Verification items for the finished model (mm, model axes). Give positions to 0.01 mm unless a question says otherwise; leave off trailing zeros. Order: outer loops, then holes, each group sorted by start corner. A loop starts at its lowest first (then second) coordinate and runs counter-clockwise, first axis right, second up. Notation, with made-up numbers: (39, 61.5) -> (55, 61.5) arc R20 cw to (55, 95.5) -> close; hole circle Ø8 at (34, 53.25). An arc over 180 degrees is marked (long way). Write each question's results on one line, items separated by ' | '. Start each with the question number.
1. Cross-section at A-A, the plane x = -25. Enter the section's corners in (y, z).
2. Cross-section at D-D, the plane y = -55. Enter the section's corners in (x, z), then the cut area to 3 significant figures.
3. Cross-section at C-C, the plane z = 3.85. State how many separate pieces and enclosed holes the cut face has, then the cut area to 3 significant figures.
4. Mould release check, pull along Y, two halves, no side actions. Record for faces 1 (the face through (-1, -75, 2)), 2 (the face through (-23.43, -0.65, 2.53)), 3 (the face through (-75, -1, 2)): +Y half, -Y half, draft (parallel to the pull), parting line (faces both ways), or undercut.
5. Material ranges on L1, parallel to Y at x = 0, z = 1.95; L2, parallel to X at y = 43, z = 3.3; L3, parallel to X at y = 44, z = 4.3, recorded low to high. Write a range as from..to.
from build123d import *

# Parameters (mm, degrees)
ESQUISSE1_W                  = 150
ESQUISSE1_H                  = 150
BOSS_EXTRU_1_DEPTH           = 5
ENL_V_MAT_EXTRU_1_DEPTH      = 5
D_GAGEMENT_M31_D             = 3.4
CONG_1_R                     = 0.5
ENL_V_MAT_EXTRU_2_REACH      = 108.184
ESQUISSE6_R                  = 2.75
R_P_TITION_CIRCULAIRE1_COUNT = 4


with BuildPart() as part:
    # Esquisse1 → Boss.-Extru.1 (new body)
    with BuildSketch(Plane.XY):
        Rectangle(ESQUISSE1_W, ESQUISSE1_H)
    extrude(amount=BOSS_EXTRU_1_DEPTH)

    # Esquisse2 → Enlèv. mat.-Extru.1 (cut)
    with BuildSketch(Plane.XY.offset(5)):
        with BuildLine():
            Line((45, 75), (75, 75))
            Line((75, 75), (75, 45))
            ThreePointArc((75, 45), (53.786796564, 53.786796564), (45, 75))
        make_face()
        with BuildLine():
            Line((75, -75), (45, -75))
            ThreePointArc((45, -75), (53.786796564, -53.786796564), (75, -45))
            Line((75, -45), (75, -75))
        make_face()
        with BuildLine():
            Line((-75, -75), (-75, -45))
            ThreePointArc((-75, -45), (-53.786796564, -53.786796564), (-45, -75))
            Line((-45, -75), (-75, -75))
        make_face()
        with BuildLine():
            Line((-75, 75), (-45, 75))
            ThreePointArc((-45, 75), (-53.786796564, 53.786796564), (-75, 45))
            Line((-75, 45), (-75, 75))
        make_face()
    extrude(amount=-ENL_V_MAT_EXTRU_1_DEPTH, mode=Mode.SUBTRACT)

    # Dégagement M31 (through all)
    with Locations(Plane(origin=(0, 0, 0), x_dir=(-1, 0, 0), z_dir=(0, 0, -1))):
        with Locations((0, 25), (0, -25), (60, 0), (25, 0), (-25, 0), (-60, 0)):
            Hole(D_GAGEMENT_M31_D / 2)

    # Congé1
    cong_1_edges = [part.edges().sort_by_distance(p)[0] for p in [
        (-75, 45, 2.5),
        (-45, 75, 2.5),
        (-45, -75, 2.5),
        (-75, -45, 2.5),
        (75, -45, 2.5),
        (45, -75, 2.5),
        (75, 45, 2.5),
        (45, 75, 2.5),
    ]]
    fillet(cong_1_edges, radius=CONG_1_R)

    # Esquisse6 → Enlèv. mat.-Extru.2 (cut, up to next)
    with BuildSketch(Plane(origin=(0, 0, 0), x_dir=(-1, 0, 0), z_dir=(0, 0, -1)), mode=Mode.PRIVATE) as enl_v_mat_extru_2_sk1:
        with Locations((-44.504098636, 44.504098636)):
            Circle(ESQUISSE6_R)
    enl_v_mat_extru_2_tool1 = extrude(enl_v_mat_extru_2_sk1.sketch, amount=-ENL_V_MAT_EXTRU_2_REACH, mode=Mode.PRIVATE) & part.part
    enl_v_mat_extru_2 = enl_v_mat_extru_2_tool1.solids().sort_by_distance((44.504099, 44.504099, 0))[0]
    add(enl_v_mat_extru_2, mode=Mode.SUBTRACT)

    # Répétition circulaire1: Enlèv. mat.-Extru.2 ×4 about axis
    r_p_tition_circulaire1_axis = Axis((-0.053962748, -0.053962748, 0), (0, 0, 1))
    for i in range(1, R_P_TITION_CIRCULAIRE1_COUNT):
        add(enl_v_mat_extru_2.rotate(r_p_tition_circulaire1_axis, i * 360 / R_P_TITION_CIRCULAIRE1_COUNT), mode=Mode.SUBTRACT)


solid = part.part
Results below:
1) outline: (-75, 0) -> (-1.7, 0) -> (-1.7, 5) -> (-75, 5) -> close; (1.7, 0) -> (75, 0) -> (75, 5) -> (1.7, 5) -> close
2) outline: (-52.64, 0) -> (52.64, 0) -> (52.64, 5) -> (-52.64, 5) -> close | area: 526 mm²
3) separate pieces: 1 | enclosed holes: 10 | area: 19,500 mm²
4) face 1: -Y half | face 2: undercut | face 3: draft
5) L1: y = -75..-26.7, -23.3..23.3, 26.7..75 | L2: x = -75..-46.91, -42.31..42.2, 46.81..75 | L3: x = -75..-47.32, -41.91..41.8, 47.21..75
